The listing builds one solid part. Answer for the finished solid, in the listing's coordinates (mm). Face numbers are marked on the shaded views. Coordinates: 2 decimals unless noted, no trailing zeros. Loops run counter-clockwise (first coordinate to the right, second up) from the corner with the lowest first, then second, coordinate; pieces in that order, holes last. Notation, with made-up numbers: (-5.5, 66) - (2.5, 66) arc R29 ccw to (2.5, 98) - close; hole circle Ø9 at (-24, -14.75). An arc over 180 degrees is marked (long way). Return JSON: item names as keys, results as strings. Group by question number.
1. Find the intervals of material crossed by line 1 along Z through (x, y) = (32, 14); line 2 along X through (y, z) = (-9, 2.5); line 3 along Y through (x, z) = (222.5, 12.75), in increasing order.
2. Section C-C (z = -4.25) is taken. Write down the section's boundary in (x, y), and give its area (3 significant figures).
3. Each of these flat-tipped pins is pushed along its axis until it touches: P1, Ø3, axis at x = 140.5, y = 81, coming from the +Z side; P2, Ø3, axis at x = 25, z = 1.5, coming from the -Y side; P3, Ø10, axis at x = 192.5, y = 23, coming from the -Z side. Where does it stop, or does it pass through?
4. Section B-B (y = 104.5) is taken. Write down the section's boundary in (x, z).
5. The mould has two halves that part along Z. Classify the marked faces 1, 2 and 3: pulls with the +Z half, pulls with the -Z half, needs draft (parallel to the pull), parting line crosses it, or undercut.
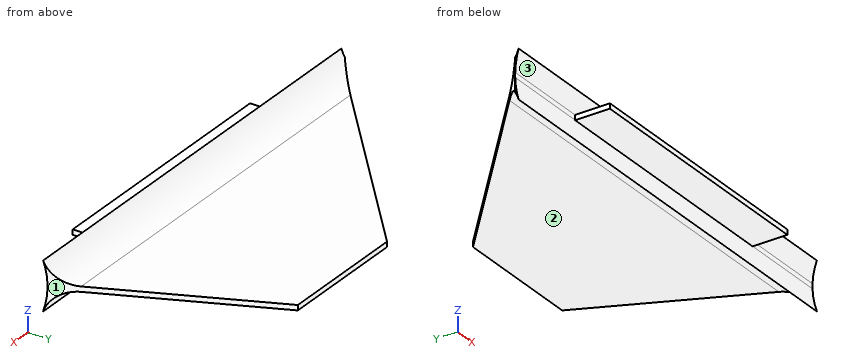
```python
from build123d import *

# Parameters (mm, degrees)
BOSS_EXTRUDE1_DEPTH = 2.9972
EXTRUDE_THIN1_REACH = 279.516
FILLET1_R           = 17.78


with BuildPart() as part:
    # Sketch1 → Boss-Extrude1 (new body)
    with BuildSketch(Plane.XY):
        Polygon((0, 0), (127, 111.76), (203.2, 111.76), (254, 0), (202.8063, 0), (202.8063, -20.32), (51.1937, -20.32), (51.1937, 0), align=None)
    extrude(amount=BOSS_EXTRUDE1_DEPTH)

    # Extrude-Thin1: up to this plane
    extrude_thin1_end = Plane(origin=(203.2, 111.76, 2.9972), z_dir=(-0.9103664774625979, -0.41380294430119924, 0))
    # Sketch2 → Extrude-Thin1 (add, up to the surface)
    with BuildSketch(Plane(origin=(0, 0, 0), x_dir=(0, 0, -1), z_dir=(1, 0, 0)), mode=Mode.PRIVATE) as extrude_thin1_sk1:
        with BuildLine():
            ThreePointArc((12.7, -2.002489682), (-1.419520366, 0.02204761), (-15.545275431, -1.958520612))
            Line((-15.545275431, -1.958520612), (-15.544573097, -1.96096158))
            ThreePointArc((-15.544573097, -1.96096158), (-1.41952432, 0.019507613), (12.69929007, -2.004928452))
            Line((12.69929007, -2.004928452), (12.7, -2.002489682))
        make_face()
    extrude_thin1_tool1 = split(extrude(extrude_thin1_sk1.sketch, amount=EXTRUDE_THIN1_REACH, mode=Mode.PRIVATE), bisect_by=extrude_thin1_end, keep=Keep.BOTH, mode=Mode.PRIVATE)
    add(extrude_thin1_tool1.solids().sort_by_distance((0, -1.92456, -12.427752))[0])

    # Fillet1
    # the kernel refuses this fillet: 17.78 mm, written as the material it adds along each edge
    with BuildSketch(Plane(origin=(0, 0, 0), x_dir=(0, 1, 0), z_dir=(1, 0, 0))) as fillet1_piece_1_section:
        with BuildLine():
            CenterArc((15.036348307, -17.78), FILLET1_R, 90, 73.398450401)
            ThreePointArc((-2.002489682, -12.7), (-0.597845135, -6.413606594), (0, 0))
            Line((0, 0), (15.036348307, 0))
        make_face()
    fillet1_piece_1 = extrude(amount=291.590870767, mode=Mode.PRIVATE)
    fillet1_piece_1 = split(fillet1_piece_1, bisect_by=Plane(origin=(74.006923082, 65.126092312, -3.495773927), z_dir=(0.6606278948920264, -0.750713516922754, 0)), keep=Keep.TOP, mode=Mode.PRIVATE)
    fillet1_piece_1 = split(fillet1_piece_1, bisect_by=Plane(origin=(230.677770328, 51.308905278, -3.495773927), z_dir=(-0.9103664774625979, -0.41380294430119924, 0)), keep=Keep.TOP, mode=Mode.PRIVATE)
    add(fillet1_piece_1)
    with BuildSketch(Plane(origin=(291.585706816, 0, 2.9972), x_dir=(0, -0.15421422141514082, 0.9880374354817341), z_dir=(-1, 0, 0))) as fillet1_piece_2_section:
        with BuildLine():
            CenterArc((15.248805398, 17.596363006), FILLET1_R, 188.871226526, 72.886892423)
            Line((-2.318500205, 14.854434149), (0, 0))
            ThreePointArc((0, 0), (6.35, 0.398437524), (12.7, 0))
        make_face()
    fillet1_piece_2 = extrude(amount=291.585706816, mode=Mode.PRIVATE)
    fillet1_piece_2 = split(fillet1_piece_2, bisect_by=Plane(origin=(74.031944404, 65.148111076, 6.44558698), z_dir=(0.6606278948920264, -0.750713516922754, 0)), keep=Keep.TOP, mode=Mode.PRIVATE)
    fillet1_piece_2 = split(fillet1_piece_2, bisect_by=Plane(origin=(230.652775468, 51.36389397, 6.44558698), z_dir=(-0.9103664774625979, -0.41380294430119924, 0)), keep=Keep.TOP, mode=Mode.PRIVATE)
    add(fillet1_piece_2)


solid = part.part
```
The answers:
{
 "1": {"line 1": "z = -0.03 to 3.03", "line 2": "x = 51.19 to 202.81", "line 3": "y = -1.24 to -0.83"},
 "2": {"outline": "(0, -0.31) - (254.14, -0.31) - (252.41, 3.5) - (3.98, 3.5) - (0, 0) - close", "area": "957 mm2"},
 "3": {"P1": "stops at z = 3", "P2": "stops at y = 0", "P3": "stops at z = 0"},
 "4": {"outline": "(118.75, 0) - (206.5, 0) - (206.5, 3) - (118.75, 3) - close"},
 "5": {"face 1": "needs draft", "face 2": "pulls with the -Z half", "face 3": "undercut"}
}
